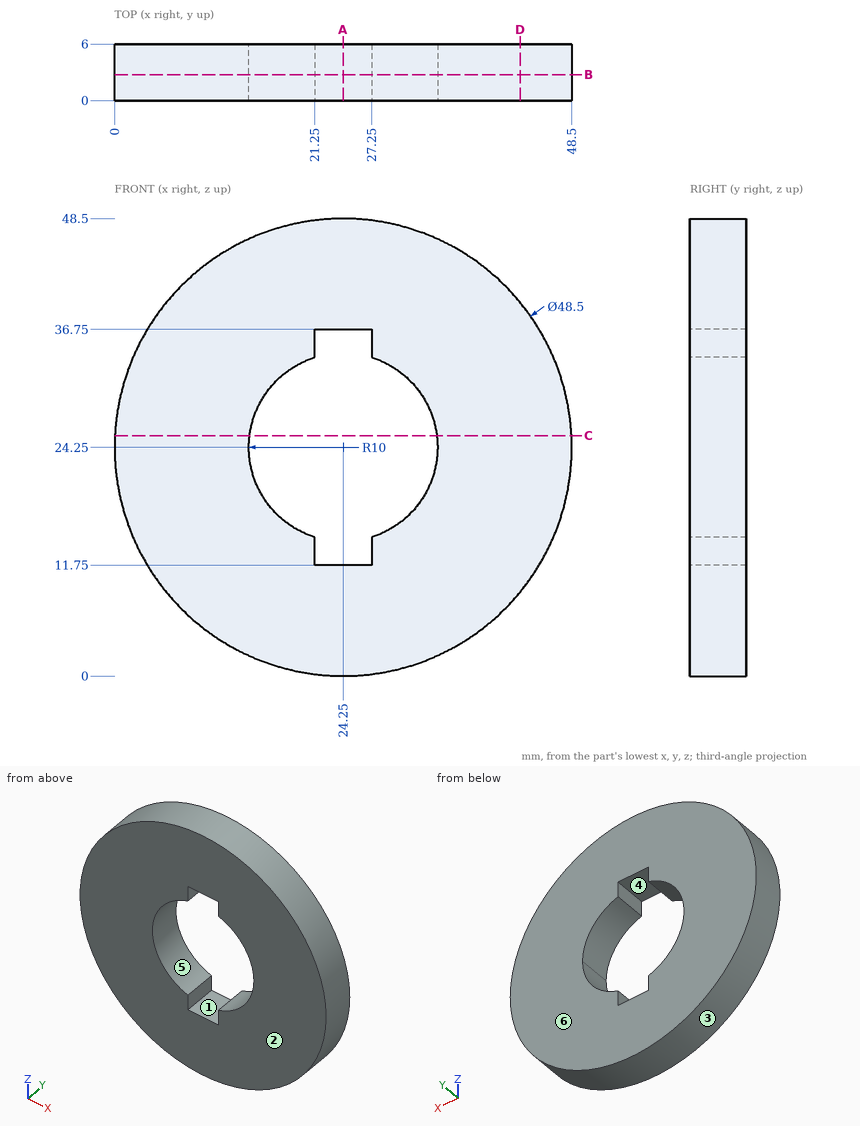
Design review of the part shown in the three views and the two pictorial views. Dimensions are in mm from the part's minimum x, y and z. A direction names the side the tool comes from. Coordinates: 2 decimals unless noted, no trailing zeros. Write each loop counter-clockwise with the first axis right and the second up, starting at its lowest first coordinate (ties: lowest second). Pieces come first, ordered by that corner, then holes. Notation, with made-up numbers: (-14.5, 68) - (8.5, 68) arc R12 cw to (8.5, 88) - close; hole circle Ø8 at (-27.5, -37.75). An arc over 180 degrees is marked (long way). Write item = value, one per line.
(1) Consider section B-B, the plane y = 2.75. Give the boundary of the cut face in (x, z).
Result sheet:
outline = circle Ø48.5 at (24.25, 24.25); hole (21.25, 11.75) - (27.25, 11.75) - (27.25, 14.71) arc R10 ccw to (34.25, 24.25) arc R10 ccw to (27.25, 33.79) - (27.25, 36.75) - (21.25, 36.75) - (21.25, 33.79) arc R10 ccw to (21.25, 14.71) - close
(2) Mouldability with a two-part tool opening along X and no side actions: class the marked faces 1, 2, 3 and 4 as pulls with the +X half, pulls with the -X half, needs draft (parallel to the pull), parting line crosses it, or undercut.
Result sheet:
face_1 = undercut
face_2 = needs draft
face_3 = parting line crosses it
face_4 = undercut
(3) For line 1 (Z direction, x = 25, y = 3.5); line 2 (X direction, y = 4.2, z = 18); line 3 (X direction, y = 0.3, z = 14), list the stretches that pass through material, from the lowest coordinate up. Write a range as [from, to].
Result sheet:
line_1 = [0.01, 11.75], [36.75, 48.49]
line_2 = [0.82, 16.44], [32.06, 47.68]
line_3 = [2.27, 21.25], [27.25, 46.23]
(4) For P1, Ø1.5, axis at y = 3, z = 35.5, coming from the +X side; P2, Ø0.9, axis at y = 3, z = 13.5, coming from the -X side; P3, Ø3, axis at x = 42.5, y = 5, coming from the -Z side, all flat-tipped, find the tip position at first contact; note any pin that passes through.
Result sheet:
P1 = 46.11
P2 = 2.3
P3 = 6.71
(5) Machinability: for the marked faces 5 and 6, which of the approach directions +Z, -Z, +X, -X, +Y, -Y give a long, thin tool a straight path to every point of the face, cutting with its end or side? Answer none if there is none.
Result sheet:
face_5 = +Y, -Y
face_6 = +Z, -Z, +X, -X, +Y
(6) Consider section A-A, the plane x = 24.25. Give the boundary of the cut face in (y, z), then the cut area to 3 significant figures.
Result sheet:
outline = (0, 0) - (6, 0) - (6, 11.75) - (0, 11.75) - close; (0, 36.75) - (6, 36.75) - (6, 48.5) - (0, 48.5) - close
area = 141 mm^2
(7) Consider section D-D, the plane x = 43. Give the boundary of the cut face in (y, z).
Result sheet:
outline = (0, 8.87) - (6, 8.87) - (6, 39.63) - (0, 39.63) - close
(8) Consider section C-C, the plane z = 25.5. Give the boundary of the cut face in (x, y), then the cut area to 3 significant figures.
Result sheet:
outline = (0.03, 0) - (14.33, 0) - (14.33, 6) - (0.03, 6) - close; (34.17, 0) - (48.47, 0) - (48.47, 6) - (34.17, 6) - close
area = 172 mm^2
